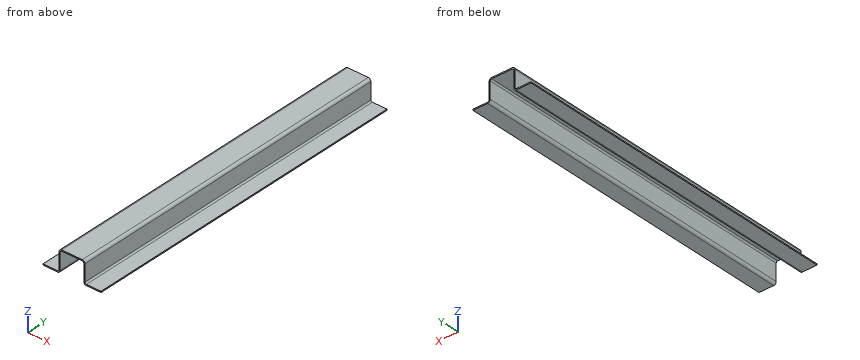
```python
from build123d import *

# Parameters (mm, degrees)
SKETCH1_W                      = 45
SKETCH1_H                      = 578
BASE_FLANGE1_DEPTH             = 2
EDGE_FLANGE1_STRIP_W           = 13
EDGE_FLANGE1_STRIP_H           = 2
EDGE_FLANGE1_STRIP_CUT_DEPTH   = 578
EDGE_FLANGE1_STRIP_2_W         = 13
EDGE_FLANGE1_STRIP_2_H         = 2
EDGE_FLANGE1_STRIP_CUT_2_DEPTH = 578
EDGE_FLANGE1_DEPTH             = 578
EDGE_FLANGE1_BEND_DEPTH        = 578
EDGE_FLANGE2_STRIP_W           = 13
EDGE_FLANGE2_STRIP_H           = 2
EDGE_FLANGE2_STRIP_CUT_DEPTH   = 578
EDGE_FLANGE2_STRIP_2_W         = 13
EDGE_FLANGE2_STRIP_2_H         = 2
EDGE_FLANGE2_STRIP_CUT_2_DEPTH = 578
EDGE_FLANGE2_DEPTH             = 578
EDGE_FLANGE2_BEND_DEPTH        = 578


# Sheet-metal steps are written as plain solids
with BuildPart() as part:
    # Sketch1 → Base-Flange1 (new body)
    with BuildSketch(Plane.XY):
        Rectangle(SKETCH1_W, SKETCH1_H)
    extrude(amount=-BASE_FLANGE1_DEPTH)

    # Edge-Flange1 strip (across the edge) → Edge-Flange1 strip cut (cut)
    with BuildSketch(Plane(origin=(22.5, 289, -2), x_dir=(-1, 0, 0), z_dir=(0, -1, 0))):
        with Locations((-2, -1)):
            Rectangle(EDGE_FLANGE1_STRIP_W, EDGE_FLANGE1_STRIP_H)
    extrude(amount=EDGE_FLANGE1_STRIP_CUT_DEPTH, mode=Mode.SUBTRACT)

    # Edge-Flange1 strip 2 (across the edge) → Edge-Flange1 strip cut 2 (cut)
    with BuildSketch(Plane(origin=(-22.5, -289, -2), x_dir=(1, 0, 0), z_dir=(0, 1, 0))):
        with Locations((-2, -1)):
            Rectangle(EDGE_FLANGE1_STRIP_2_W, EDGE_FLANGE1_STRIP_2_H)
    extrude(amount=EDGE_FLANGE1_STRIP_CUT_2_DEPTH, mode=Mode.SUBTRACT)

    # Edge-Flange1 section (across the edge) → Edge-Flange1 (add)
    with BuildSketch(Plane(origin=(22.5, 289, -2), x_dir=(-1, 0, 0), z_dir=(0, -1, 0))):
        with BuildLine():
            Line((0, 2.5), (0, 36))
            Line((0, 36), (2, 36))
            Line((2, 36), (2, 2.5))
            ThreePointArc((2, 2.5), (2.732233047, 0.732233047), (4.5, 0))
            Line((4.5, 0), (4.5, -2))
            ThreePointArc((4.5, -2), (1.318019485, -0.681980515), (0, 2.5))
        make_face()
    extrude(amount=EDGE_FLANGE1_DEPTH)

    # Edge-Flange1 section 2 (across the edge) → Edge-Flange1 bend (add)
    with BuildSketch(Plane(origin=(-22.5, -289, -2), x_dir=(1, 0, 0), z_dir=(0, 1, 0))):
        with BuildLine():
            Line((0, 2.5), (0, 36))
            Line((0, 36), (2, 36))
            Line((2, 36), (2, 2.5))
            ThreePointArc((2, 2.5), (2.732233047, 0.732233047), (4.5, 0))
            Line((4.5, 0), (4.5, -2))
            ThreePointArc((4.5, -2), (1.318019485, -0.681980515), (0, 2.5))
        make_face()
    extrude(amount=EDGE_FLANGE1_BEND_DEPTH)

    # Edge-Flange2 strip (across the edge) → Edge-Flange2 strip cut (cut)
    with BuildSketch(Plane(origin=(-22.5, 289, -38), x_dir=(0, 0, 1), z_dir=(0, -1, 0))):
        with Locations((-2, -1)):
            Rectangle(EDGE_FLANGE2_STRIP_W, EDGE_FLANGE2_STRIP_H)
    extrude(amount=EDGE_FLANGE2_STRIP_CUT_DEPTH, mode=Mode.SUBTRACT)

    # Edge-Flange2 strip 2 (across the edge) → Edge-Flange2 strip cut 2 (cut)
    with BuildSketch(Plane(origin=(22.5, -289, -38), x_dir=(0, 0, 1), z_dir=(0, 1, 0))):
        with Locations((-2, -1)):
            Rectangle(EDGE_FLANGE2_STRIP_2_W, EDGE_FLANGE2_STRIP_2_H)
    extrude(amount=EDGE_FLANGE2_STRIP_CUT_2_DEPTH, mode=Mode.SUBTRACT)

    # Edge-Flange2 section (across the edge) → Edge-Flange2 (add)
    with BuildSketch(Plane(origin=(-22.5, 289, -38), x_dir=(0, 0, 1), z_dir=(0, -1, 0))):
        with BuildLine():
            Line((0, 2.5), (0, 28))
            Line((0, 28), (2, 28))
            Line((2, 28), (2, 2.5))
            ThreePointArc((2, 2.5), (2.732233047, 0.732233047), (4.5, 0))
            Line((4.5, 0), (4.5, -2))
            ThreePointArc((4.5, -2), (1.318019485, -0.681980515), (0, 2.5))
        make_face()
    extrude(amount=EDGE_FLANGE2_DEPTH)

    # Edge-Flange2 section 2 (across the edge) → Edge-Flange2 bend (add)
    with BuildSketch(Plane(origin=(22.5, -289, -38), x_dir=(0, 0, 1), z_dir=(0, 1, 0))):
        with BuildLine():
            Line((0, 2.5), (0, 28))
            Line((0, 28), (2, 28))
            Line((2, 28), (2, 2.5))
            ThreePointArc((2, 2.5), (2.732233047, 0.732233047), (4.5, 0))
            Line((4.5, 0), (4.5, -2))
            ThreePointArc((4.5, -2), (1.318019485, -0.681980515), (0, 2.5))
        make_face()
    extrude(amount=EDGE_FLANGE2_BEND_DEPTH)


solid = part.part
```
Read the model definition and answer for the solid it produces. Units are mm, in the model's axes. Give positions to 0.01 mm unless a question says otherwise; leave off trailing zeros. Order: outer loops, then holes, each group sorted by start corner. A loop starts at its lowest first (then second) coordinate and runs counter-clockwise, first axis right, second up.
(1) Straight lines are drawn through the part: L1, parallel to X at y = 124, z = -21; L2, parallel to X at y = 246.5, z = -4; L3, parallel to Z at x = -17, y = 177.5. For each, find the intervals that lie inside material, in ascending order.
(2) Find section A-A (z = -14.5). Give the vertices of the cut face in (x, y), plus the area to 3 significant figures.
(3) Given pin 1 (14.5 mm diameter, centred on y = 36, z = -24, fed in from -X); pin 2 (12 mm diameter, centred on x = 12.5, y = -137.5, fed in from +Z); pin 3 (13 mm diameter, centred on x = 34, y = 104, fed in from +Z); pin 4 (6 mm diameter, centred on x = -24.5, y = -138, fed in from +Z), each flat-ended and moving along its own axis, determine where each tip first touches the part or whether it passes through.
(4) Find section C-C (x = -43.5). Give the vertices of the cut face in (y, z).
(5) Find section B-B (y = -242.5). Give the vertices of the cut face in (x, z).
Result sheet:
1. L1: x = -22.5 to -20.5, 20.5 to 22.5
1. L2: x = -22.47 to -20.45, 20.45 to 22.47
1. L3: z = -2 to 0
2. outline: (-22.5, -289) - (-20.5, -289) - (-20.5, 289) - (-22.5, 289) - close; (20.5, -289) - (22.5, -289) - (22.5, 289) - (20.5, 289) - close
2. area: 2,310 mm2
3. pin 1: stops at x = -22.5
3. pin 2: stops at z = 0
3. pin 3: stops at z = -36
3. pin 4: stops at z = -1.67
4. outline: (-289, -38) - (289, -38) - (289, -36) - (-289, -36) - close
5. outline: (-50.5, -38) - (-25, -38) arc R4.5 ccw to (-20.5, -33.5) - (-20.5, -4.5) arc R2.5 cw to (-18, -2) - (18, -2) arc R2.5 cw to (20.5, -4.5) - (20.5, -33.5) arc R4.5 ccw to (25, -38) - (50.5, -38) - (50.5, -36) - (25, -36) arc R2.5 cw to (22.5, -33.5) - (22.5, -4.5) arc R4.5 ccw to (18, 0) - (-18, 0) arc R4.5 ccw to (-22.5, -4.5) - (-22.5, -33.5) arc R2.5 cw to (-25, -36) - (-50.5, -36) - close
